from build123d import *

# Parameters (mm, degrees)
SKETCH1_R           = 15.08125
BOSS_EXTRUDE1_DEPTH = 3.175
FILLET1_R           = 12.7


with BuildPart() as part:
    # Sketch1 → Boss-Extrude1 (new body)
    with BuildSketch(Plane(origin=(0, 0, 0), x_dir=(0, 0, -1), z_dir=(1, 0, 0))):
        with BuildLine():
            Line((-558.8, 609.6), (-558.8, 685.8))
            Line((-558.8, 685.8), (558.8, 685.8))
            Line((558.8, 685.8), (558.8, 609.6))
            ThreePointArc((558.8, 609.6), (492.779998657, 429.230002015), (325.91999876, 334.100000517))
            Line((325.91999876, 334.100000517), (152.4, 304.8))
            Line((152.4, 304.8), (-152.4, 304.8))
            Line((-152.4, 304.8), (-325.91999876, 334.100000517))
            ThreePointArc((-325.91999876, 334.100000517), (-492.779998657, 429.230002015), (-558.8, 609.6))
        make_face()
        with Locations((-508, 647.7)):
            Circle(SKETCH1_R, mode=Mode.SUBTRACT)
        with Locations((508, 647.7)):
            Circle(SKETCH1_R, mode=Mode.SUBTRACT)
    extrude(amount=BOSS_EXTRUDE1_DEPTH)

    # Fillet1
    fillet1_edges = [part.edges().sort_by_distance(p)[0] for p in [
        (1.5875, 304.8, -152.4),
        (1.5875, 304.8, 152.4),
        (1.5875, 685.8, 558.8),
        (1.5875, 685.8, -558.8),
    ]]
    fillet(fillet1_edges, radius=FILLET1_R)


solid = part.part
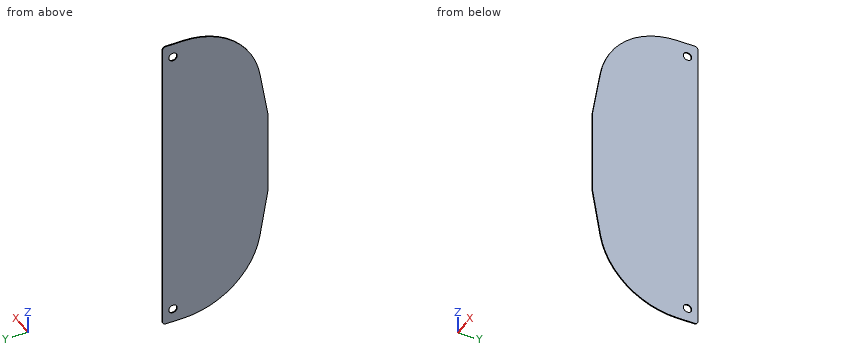
The listing builds one solid part. Answer for the finished solid, in the listing's coordinates (mm). Give positions to 0.01 mm unless a question says otherwise; leave off trailing zeros. Loops run counter-clockwise (first coordinate to the right, second up) from the corner with the lowest first, then second, coordinate; pieces in that order, holes last. Notation, with made-up numbers: (9, -18.5) - (57, -18.5) arc R36 cw to (57, 20.5) - close; hole circle Ø7 at (-24, 13.25). An arc over 180 degrees is marked (long way). Use one line per item in the form item = value.
1. Section A-A on y = 647.7 is taken. Give the vertices of the cut face in (x, z) (3 decimals), then the cut area to 3 significant figures.
Calculated:
outline = (0, -558.8) - (3.175, -558.8) - (3.175, -523.081) - (0, -523.081) - close; (0, -492.919) - (3.175, -492.919) - (3.175, 492.919) - (0, 492.919) - close; (0, 523.081) - (3.175, 523.081) - (3.175, 558.8) - (0, 558.8) - close
area = 3,360 mm^2
2. Section D-D on z = -449 is taken. Give the vertices of the cut face in (x, y) (3 decimals), then the cut area to 3 significant figures.
Calculated:
outline = (0, 387.564) - (3.175, 387.564) - (3.175, 685.8) - (0, 685.8) - close
area = 947 mm^2
3. Section C-C on x = 0.7 is taken. Give the vertices of the cut face in (y, z).
Calculated:
outline = (304.8, -151.34) arc R12.7 ccw to (304.98, -153.45) - (334.1, -325.92) arc R279.4 ccw to (609.6, -558.8) - (673.1, -558.8) arc R12.7 ccw to (685.8, -546.1) - (685.8, 546.1) arc R12.7 ccw to (673.1, 558.8) - (609.6, 558.8) arc R279.4 ccw to (334.1, 325.92) - (304.98, 153.45) arc R12.7 ccw to (304.8, 151.34) - close; hole circle Ø30.16 at (647.7, -508); hole circle Ø30.16 at (647.7, 508)
4. Given pin 1 Ø1 at (x, y) = (0.5, 499.5) entering from -Z; pin 2 Ø2 at (y, z) = (399.5, 363) entering from -X; pin 3 Ø18 at (y, z) = (647.7, 508) entering from +X, each flat-ended and moving along its own axis, determine where each tip first touches the part or whether it passes through.
Calculated:
pin_1 = -536.41
pin_2 = 0
pin_3 = through
5. Section B-B on z = 508 is taken. Give the vertices of the cut face in (x, y) (3 decimals).
Calculated:
outline = (0, 448.956) - (3.175, 448.956) - (3.175, 632.619) - (0, 632.619) - close; (0, 662.781) - (3.175, 662.781) - (3.175, 685.8) - (0, 685.8) - close
6. Find the intervals of material crossed by line 1 along Z through (x, y) = (0.95, 647.7); line 2 along Y through (x, z) = (0.95, -508); line 3 along Y through (x, z) = (2.8, -230.5), in increasing order. Write a range as [from, to].
Calculated:
line_1 = [-558.8, -523.08], [-492.92, 492.92], [523.08, 558.8]
line_2 = [448.96, 632.62], [662.78, 685.8]
line_3 = [317.99, 685.8]
